The drawing under review shows one solid part. Ordinate dimensions are in mm from its lowest x, y, z. A direction names the side the tool comes from. Coordinates: 2 decimals unless noted, no trailing zeros. Order: outer loops, then holes, each group sorted by start corner. A loop starts at its lowest first (then second) coordinate and runs counter-clockwise, first axis right, second up. Notation, with made-up numbers: (39.25, 73) - (68.25, 73) arc R30 ccw to (68.25, 98) - close; hole circle Ø3 at (38, 55). An arc over 180 degrees is marked (long way). Answer in a Markdown table with one row per item.
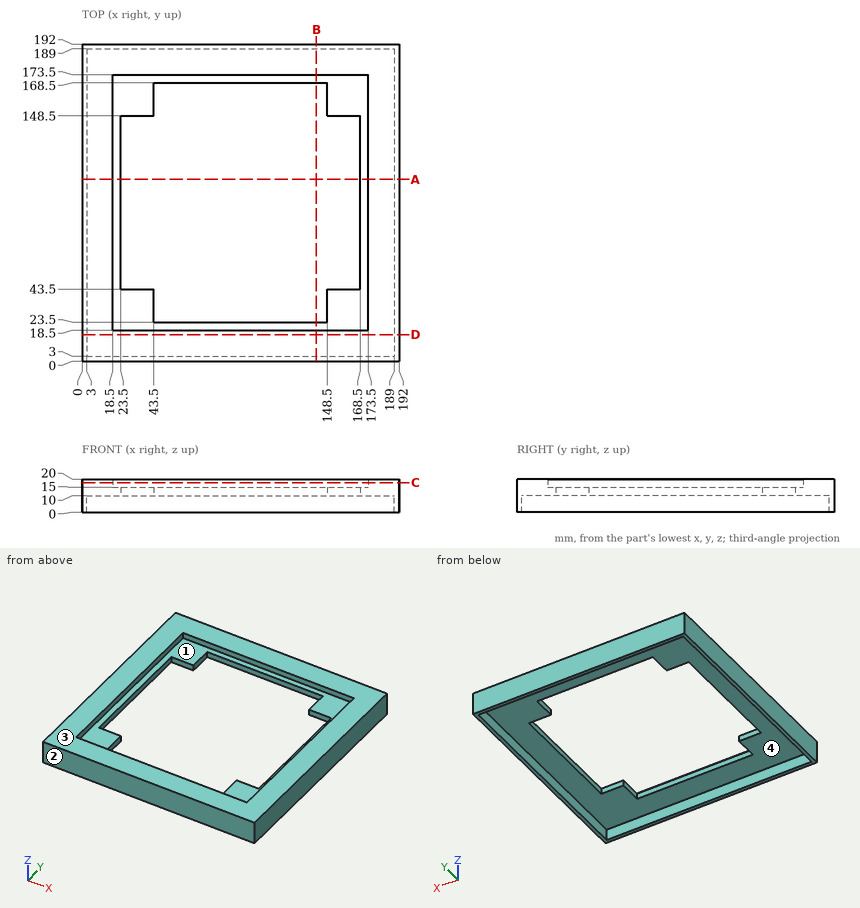
Item 1: Mouldability with a two-part tool opening along X and no side actions: class the marked faces 3 and 4 as +X half, -X half, draft (parallel to the pull), parting line (faces both ways), or undercut.
Check values:
| item | result |
|---|---|
| face 3 | draft |
| face 4 | undercut |
Item 2: To check wall thickness, follow line 1 (Y direction, x = 164, z = 15.5); line 2 (X direction, y = 36, z = 9). State the ranges of each line that lie inside material, in increasing order. Write a range as from..to.
Check values:
| item | result |
|---|---|
| line 1 | 0..18.5, 173.5..192 |
| line 2 | 0..3, 189..192 |
Item 3: Clearance check with a flat-ended pin moving along its axis: pin 1 Ø1.5 at (x, y) = (110.5, 169) entering from +Z. State where the tip first meets the part, or that it passes through.
Check values:
| item | result |
|---|---|
| pin 1 | z = 15 |
Item 4: Tool access review of the marked faces 1 and 2: name each direction out of +Z, -Z, +X, -X, +Y, -Y from which nothing blocks a thin tool from reaching the whole face with its end or side.
Check values:
| item | result |
|---|---|
| face 1 | +Z |
| face 2 | +Z, -Z, +X, -X, -Y |
Item 5: We need section C-C, the plane z = 17.75. Write out the cut boundary in (x, y), then the cut area to 3 significant figures.
Check values:
| item | result |
|---|---|
| outline | (0, 0) - (192, 0) - (192, 192) - (0, 192) - close; hole (18.5, 18.5) - (173.5, 18.5) - (173.5, 173.5) - (18.5, 173.5) - close |
| area | 12,800 mm^2 |
Item 6: We need section D-D, the plane y = 16. Write out the cut boundary in (x, z).
Check values:
| item | result |
|---|---|
| outline | (0, 0) - (3, 0) - (3, 10) - (189, 10) - (189, 0) - (192, 0) - (192, 20) - (0, 20) - close |
Item 7: We need section A-A, the plane y = 110. Write out the cut boundary in (x, z).
Check values:
| item | result |
|---|---|
| outline | (0, 0) - (3, 0) - (3, 10) - (23.5, 10) - (23.5, 15) - (18.5, 15) - (18.5, 20) - (0, 20) - close; (168.5, 10) - (189, 10) - (189, 0) - (192, 0) - (192, 20) - (173.5, 20) - (173.5, 15) - (168.5, 15) - close |
